from build123d import *

# Parameters (mm, degrees)
BOSS_EXTRUDE1_DEPTH   = 0.3
EXTRUDE_THIN1_DEPTH   = 5
EXTRUDE_THIN1_2_DEPTH = 0.3
EXTRUDE_THIN1_START   = 4.7
EXTRUDE_THIN1_3_DEPTH = 0.3
FILLET2_R             = 0.3
CUT_EXTRUDE2_REACH    = 8.308
SKETCH5_W             = 1
SKETCH5_H             = 0.5
SKETCH6_W             = 0.7
SKETCH6_H             = 0.4
SKETCH6_W_2           = 0.5
SKETCH6_H_2           = 0.8
CUT_EXTRUDE3_DEPTH    = 0.2
CUT_EXTRUDE4_DEPTH    = 0.1
BOSS_EXTRUDE2_DEPTH   = 3
CHAMFER1_SIZE         = 0.2
SKETCH9_W             = 0.7
SKETCH9_H             = 0.4
BOSS_EXTRUDE3_DEPTH   = 1
SKETCH10_W            = 0.3
SKETCH10_H            = 0.2
CUT_EXTRUDE5_DEPTH    = 0.3
SKETCH11_R            = 0.07
CUT_EXTRUDE6_DEPTH    = 1


# Read off the part's stored shape, not the designer's step: Extrude-Thin1
with BuildPart() as part:
    # Sketch2 → Boss-Extrude1 (new body)
    with BuildSketch(Plane(origin=(0, 0, 0), x_dir=(1, 0, 0), z_dir=(0, 1, 0))):
        with BuildLine():
            Line((-2.257247878, 1.145651273), (-0.514495755, 2.191302547))
            ThreePointArc((-0.514495755, 2.191302547), (0, 2.333809621), (0.514495755, 2.191302547))
            Line((0.514495755, 2.191302547), (2.257247878, 1.145651273))
            ThreePointArc((2.257247878, 1.145651273), (2.435099953, 0.963254218), (2.5, 0.716904811))
            Line((2.5, 0.716904811), (2.5, -0.5))
            ThreePointArc((2.5, -0.5), (2.353553391, -0.853553391), (2, -1))
            Line((2, -1), (-2, -1))
            ThreePointArc((-2, -1), (-2.353553391, -0.853553391), (-2.5, -0.5))
            Line((-2.5, -0.5), (-2.5, 0.716904811))
            ThreePointArc((-2.5, 0.716904811), (-2.435099953, 0.963254218), (-2.257247878, 1.145651273))
        make_face()
    extrude(amount=BOSS_EXTRUDE1_DEPTH)

    # Extrude-Thin1 outline → Extrude-Thin1 (add)
    with BuildSketch(Plane(origin=(0, 0.3, 0), x_dir=(1, 0, 0), z_dir=(0, 1, 0))):
        with BuildLine():
            ThreePointArc((-1.8, 1.2), (-2.012132034, 1.112132034), (-2.1, 0.9))
            Line((-2.1, 0.9), (-2.1, -0.4))
            ThreePointArc((-2.1, -0.4), (-2.012132034, -0.612132034), (-1.8, -0.7))
            Line((-1.8, -0.7), (1.8, -0.7))
            ThreePointArc((1.8, -0.7), (2.012132034, -0.612132034), (2.1, -0.4))
            Line((2.1, -0.4), (2.1, 0.9))
            ThreePointArc((2.1, 0.9), (2.012132034, 1.112132034), (1.8, 1.2))
            Line((1.8, 1.2), (-1.8, 1.2))
        make_face()
        with BuildLine():
            Line((-2, -0.4), (-2, 0.9))
            ThreePointArc((-2, 0.9), (-1.941421356, 1.041421356), (-1.8, 1.1))
            Line((-1.8, 1.1), (1.8, 1.1))
            ThreePointArc((1.8, 1.1), (1.941421356, 1.041421356), (2, 0.9))
            Line((2, 0.9), (2, -0.4))
            ThreePointArc((2, -0.4), (1.941421356, -0.541421356), (1.8, -0.6))
            Line((1.8, -0.6), (-1.8, -0.6))
            ThreePointArc((-1.8, -0.6), (-1.941421356, -0.541421356), (-2, -0.4))
        make_face(mode=Mode.SUBTRACT)
    extrude(amount=EXTRUDE_THIN1_DEPTH)

    # Extrude-Thin1 2 outline → Extrude-Thin1 2 (add)
    with BuildSketch(Plane(origin=(0, 0.3, 0), x_dir=(1, 0, 0), z_dir=(0, 1, 0))):
        with BuildLine():
            ThreePointArc((-1.8, 1.1), (-1.941421356, 1.041421356), (-2, 0.9))
            Line((-2, 0.9), (-2, -0.4))
            ThreePointArc((-2, -0.4), (-1.941421356, -0.541421356), (-1.8, -0.6))
            Line((-1.8, -0.6), (1.8, -0.6))
            ThreePointArc((1.8, -0.6), (1.941421356, -0.541421356), (2, -0.4))
            Line((2, -0.4), (2, 0.9))
            ThreePointArc((2, 0.9), (1.941421356, 1.041421356), (1.8, 1.1))
            Line((1.8, 1.1), (-1.8, 1.1))
        make_face()
    extrude(amount=EXTRUDE_THIN1_2_DEPTH)

    # Extrude-Thin1 3 outline → Extrude-Thin1 3 (add)
    with BuildSketch(Plane(origin=(0, 0.3, 0), x_dir=(1, 0, 0), z_dir=(0, 1, 0)).offset(EXTRUDE_THIN1_START)):
        with BuildLine():
            ThreePointArc((-1.8, 1.1), (-1.941421356, 1.041421356), (-2, 0.9))
            Line((-2, 0.9), (-2, -0.4))
            ThreePointArc((-2, -0.4), (-1.941421356, -0.541421356), (-1.8, -0.6))
            Line((-1.8, -0.6), (1.8, -0.6))
            ThreePointArc((1.8, -0.6), (1.941421356, -0.541421356), (2, -0.4))
            Line((2, -0.4), (2, 0.9))
            ThreePointArc((2, 0.9), (1.941421356, 1.041421356), (1.8, 1.1))
            Line((1.8, 1.1), (-1.8, 1.1))
        make_face()
    extrude(amount=EXTRUDE_THIN1_3_DEPTH)

    # Fillet2
    fillet2_edges = [part.edges().sort_by_distance(p)[0] for p in [
        (2.1, 5.3, -0.25),
        (2.012132034, 5.3, -1.112132034),
        (0, 5.3, -1.2),
        (-2.012132034, 5.3, -1.112132034),
        (-2.1, 5.3, -0.25),
        (-2.012132034, 5.3, 0.612132034),
        (0, 5.3, 0.7),
        (2.012132034, 5.3, 0.612132034),
    ]]
    fillet(fillet2_edges, radius=FILLET2_R)

    # Sketch5 → Cut-Extrude2 (cut, up to next)
    with BuildSketch(Plane(origin=(0, 5.3, 0), x_dir=(1, 0, 0), z_dir=(0, 1, 0)), mode=Mode.PRIVATE) as cut_extrude2_sk1:
        with Locations((0, 0.15)):
            Rectangle(SKETCH5_W, SKETCH5_H)
    cut_extrude2_tool1 = extrude(cut_extrude2_sk1.sketch, amount=-CUT_EXTRUDE2_REACH, mode=Mode.PRIVATE) & part.part
    add(cut_extrude2_tool1.solids().sort_by_distance((0, 5.3, -0.15))[0], mode=Mode.SUBTRACT)

    # Sketch6 → Cut-Extrude3 (cut)
    with BuildSketch(Plane.XZ):
        with Locations((-1.35, 0)):
            Rectangle(SKETCH6_W, SKETCH6_H)
        with Locations((1.35, 0)):
            Rectangle(SKETCH6_W, SKETCH6_H)
        with Locations((0, -1.7)):
            Rectangle(SKETCH6_W_2, SKETCH6_H_2)
    extrude(amount=-CUT_EXTRUDE3_DEPTH, mode=Mode.SUBTRACT)

    # Sketch7 → Cut-Extrude4 (cut)
    with BuildSketch(Plane.XZ):
        with BuildLine():
            Line((-1.9, 0.9), (1.9, 0.9))
            ThreePointArc((1.9, 0.9), (2.253553391, 0.753553391), (2.4, 0.4))
            Line((2.4, 0.4), (2.4, -0.680159029))
            ThreePointArc((2.4, -0.680159029), (2.335099953, -0.926508436), (2.157247878, -1.108905491))
            Line((2.157247878, -1.108905491), (0.514495755, -2.094556765))
            ThreePointArc((0.514495755, -2.094556765), (0, -2.237063839), (-0.514495755, -2.094556765))
            Line((-0.514495755, -2.094556765), (-2.157247878, -1.108905491))
            ThreePointArc((-2.157247878, -1.108905491), (-2.335099953, -0.926508436), (-2.4, -0.680159029))
            Line((-2.4, -0.680159029), (-2.4, 0.4))
            ThreePointArc((-2.4, 0.4), (-2.253553391, 0.753553391), (-1.9, 0.9))
        make_face()
        with BuildLine():
            Line((-1.6, 0.7), (1.6, 0.7))
            ThreePointArc((1.6, 0.7), (1.953553391, 0.553553391), (2.1, 0.2))
            Line((2.1, 0.2), (2.1, -0.7))
            ThreePointArc((2.1, -0.7), (1.953553391, -1.053553391), (1.6, -1.2))
            Line((1.6, -1.2), (-1.6, -1.2))
            ThreePointArc((-1.6, -1.2), (-1.953553391, -1.053553391), (-2.1, -0.7))
            Line((-2.1, -0.7), (-2.1, 0.2))
            ThreePointArc((-2.1, 0.2), (-1.953553391, 0.553553391), (-1.6, 0.7))
        make_face(mode=Mode.SUBTRACT)
    extrude(amount=-CUT_EXTRUDE4_DEPTH, mode=Mode.SUBTRACT)

    # Sketch8 → Boss-Extrude2 (add)
    with BuildSketch(Plane.XZ.offset(-0.2)):
        Polygon((0.25, -1.46), (0.07, -1.46), (0.07, -1.62), (0.25, -1.62), (0.25, -1.78), (0.07, -1.78), (0.07, -1.94), (0.25, -1.94), (0.25, -2.1), (-0.25, -2.1), (-0.25, -1.94), (-0.07, -1.94), (-0.07, -1.78), (-0.25, -1.78), (-0.25, -1.62), (-0.07, -1.62), (-0.07, -1.46), (-0.25, -1.46), (-0.25, -1.3), (0.25, -1.3), align=None)
    extrude(amount=BOSS_EXTRUDE2_DEPTH)

    # Chamfer1
    # the kernel refuses this chamfer: 0.2 mm, written as the material it takes off along each edge
    with BuildSketch(Plane(origin=(-0.25, -2.8, -1.974336598), x_dir=(-0.027495876610586223, 0.9996219169112966, 0), z_dir=(0, 0, 1)), Plane(origin=(-0.25, -2.8, -2.294336598), x_dir=(-0.027495876610586223, 0.9996219169112966, 0), z_dir=(0, 0, 1)), Plane(origin=(-0.25, -2.8, -2.614336598), x_dir=(-0.027495876610586355, 0.9996219169112966, 0), z_dir=(0, 0, 1)), Plane(origin=(0.25, -2.8, -1.425663402), x_dir=(0.027495876610586223, 0.9996219169112966, 0), z_dir=(0, 0, -1)), Plane(origin=(0.25, -2.8, -1.105663402), x_dir=(0.027495876610586223, 0.9996219169112966, 0), z_dir=(0, 0, -1)), Plane(origin=(0.25, -2.8, -0.785663402), x_dir=(0.027495876610586223, 0.9996219169112966, 0), z_dir=(0, 0, -1))) as chamfer1_piece_1:
        Polygon((CHAMFER1_SIZE * 0.999621916911, -CHAMFER1_SIZE * 0.0274958766106), (-CHAMFER1_SIZE * 0.0274958766106, -CHAMFER1_SIZE * 0.999621916911), (0, 0), align=None)
    extrude(amount=1.188673195, mode=Mode.SUBTRACT)

    # Sketch9 → Boss-Extrude3 (add)
    with BuildSketch(Plane.XZ.offset(-0.2)):
        with Locations((1.35, 0)):
            Rectangle(SKETCH9_W, SKETCH9_H)
    boss_extrude3 = extrude(amount=BOSS_EXTRUDE3_DEPTH)

    # Sketch10 → Cut-Extrude5 (cut)
    with BuildSketch(Plane.XZ.offset(0.8)):
        with Locations((1.35, 0)):
            Rectangle(SKETCH10_W, SKETCH10_H)
        with Locations((-1.35, 0)):
            Rectangle(SKETCH10_W, SKETCH10_H)
    cut_extrude5 = extrude(amount=-CUT_EXTRUDE5_DEPTH, mode=Mode.SUBTRACT)

    # Sketch11 → Cut-Extrude6 (cut)
    with BuildSketch(Plane.XZ.offset(0.5)):
        with Locations(Location((1.35, 0, 0), (0, 0, 270))):
            Circle(SKETCH11_R)
    cut_extrude6 = extrude(amount=-CUT_EXTRUDE6_DEPTH, mode=Mode.SUBTRACT)

    # Mirror2: Boss-Extrude3, Cut-Extrude5, Cut-Extrude6 across plane
    add(boss_extrude3.mirror(Plane(origin=(0, 0, 0), x_dir=(0, 0, 1), z_dir=(1, 0, 0))))
    add(cut_extrude5.mirror(Plane(origin=(0, 0, 0), x_dir=(0, 0, 1), z_dir=(1, 0, 0))), mode=Mode.SUBTRACT)
    add(cut_extrude6.mirror(Plane(origin=(0, 0, 0), x_dir=(0, 0, 1), z_dir=(1, 0, 0))), mode=Mode.SUBTRACT)


solid = part.part
The model under review builds one solid part; all positions refer to its coordinate system, in mm. A direction names the side the tool comes from. Round coordinates to 2 decimals unless told otherwise and drop trailing zeros. Loops run counter-clockwise (first coordinate to the right, second up) from the corner with the lowest first, then second, coordinate; pieces in that order, holes last. Notation, with made-up numbers: M -37,68.25 L -1,68.25 A17 ccw -1,98.25 Z; hole C -5,66.25 d2. An arc over 180 degrees is marked long. Answer as CSV lines item,"result". Start each with the question number.
Item 1: Consider section A-A (y = 1.75). Write out the cut boundary in (x, z), then the cut area to 3 significant figures.
Item 2: Mouldability with a two-part tool opening along Y and no side actions: class faces 3 (the face through (-0.03, 5.3, -0.55)), 4 (the face through (0, 5, -0.6)) as released by +Y, released by -Y, zero draft, split by the parting line, or undercut.
Item 3: Consider section B-B (y = -2.25). Write out the cut boundary in (x, z), then the cut area to 3 significant figures.
Item 4: Wall thickness on line 1 (Y direction, x = -0.3, z = -0.8); line 2 (Z direction, x = -0.7, y = 0.5); line 3 (Y direction, x = -0.7, z = -1.55): over which ranges is each line inside the solid? List them lowest first. Write a range as [from, to].
Item 5: Consider section C-C (x = -1.1). Write out the cut boundary in (y, z), then the cut area to 3 significant figures.
Item 6: Insertion check: P1, Ø1, axis at y = 2, z = -0.5, coming from the +X side; P2, Ø1.5, axis at x = -0.5, z = 0, coming from the -Y side; P3, Ø0.8, axis at x = 1, y = 0, coming from the -Z side. Each pin has a flat end and moves straight along its axis. Give the tip position at first contact, or say it passes through.
Item 7: For faces 1 (the face through (0, 0.6, 0)), 2 (the face through (-0.5, 0.3, -1.4)), list the 3-axis set-ups (+Z, -Z, +X, -X, +Y, -Y) from which the entire face can be reached by the end or side of a thin tool; tool diameter is ignored.
Answer:
1,outline,"M -2.1,-0.9 A0.3 ccw -1.8,-1.2 L 1.8,-1.2 A0.3 ccw 2.1,-0.9 L 2.1,0.4 A0.3 ccw 1.8,0.7 L -1.8,0.7 A0.3 ccw -2.1,0.4 Z; hole M -2,-0.9 A0.2 ccw -1.8,-1.1 L 1.8,-1.1 A0.2 ccw 2,-0.9 L 2,0.4 A0.2 ccw 1.8,0.6 L -1.8,0.6 A0.2 ccw -2,0.4 Z"
1,area,"1.14 mm^2"
2,face 3,"released by +Y"
2,face 4,"undercut"
3,outline,"M -0.25,-2.1 L 0.25,-2.1 L 0.25,-1.94 L 0.07,-1.94 L 0.07,-1.78 L 0.25,-1.78 L 0.25,-1.62 L 0.07,-1.62 L 0.07,-1.46 L 0.25,-1.46 L 0.25,-1.3 L -0.25,-1.3 L -0.25,-1.46 L -0.07,-1.46 L -0.07,-1.62 L -0.25,-1.62 L -0.25,-1.78 L -0.07,-1.78 L -0.07,-1.94 L -0.25,-1.94 Z"
3,area,"0.285 mm^2"
4,line 1,"y = [0, 0.6], [5, 5.3]"
4,line 2,"z = [-1.2, 0.7]"
4,line 3,"y = [0.1, 0.3]"
5,outline,"M -0.8,-0.2 L 0,-0.2 L 0,-1.2 L 0.1,-1.2 L 0.1,-1.74 L 0,-1.74 L 0,-1.84 L 0.3,-1.84 L 0.3,-1.2 L 5,-1.2 A0.3 ccw 5.3,-0.9 L 5.3,0.4 A0.3 ccw 5,0.7 L 0.3,0.7 L 0.3,1 L 0,1 L 0,0.9 L 0.1,0.9 L 0.1,0.7 L 0,0.7 L 0,0.2 L -0.8,0.2 Z; hole M 0.6,-1.1 L 5,-1.1 L 5,0.6 L 0.6,0.6 Z"
5,area,"3.08 mm^2"
6,P1,"stops at x = 2.1"
6,P2,"stops at y = -0.8"
6,P3,"stops at z = -2.14"
7,face 1,"none"
7,face 2,"+Y"
